```python
from build123d import *

# Parameters (mm, degrees)
PAD_DEPTH       = 12
POCKET_DEPTH    = 9
SKETCH002_R     = 2.1
POCKET001_DEPTH = 3
SKETCH003_R     = 1.6
POCKET002_DEPTH = 3.001
SKETCH004_R     = 3.2
POCKET003_DEPTH = 1


with BuildPart() as part:
    # Sketch → Pad (new body)
    with BuildSketch(Plane.XY):
        with BuildLine():
            ThreePointArc((10.4, 0), (0, 10.4), (-10.4, 0))
            Line((-10.4, 0), (-22.4, 0))
            Line((-22.4, 0), (-22.4, 3))
            Line((-22.4, 3), (-13.059862, 3))
            ThreePointArc((-4, 12.789058), (-9.834436, 9.10186), (-13.059862, 3))
            Line((-4, 12.789058), (-4, 22.789058))
            Line((-4, 22.789058), (4, 22.789058))
            Line((4, 22.789058), (4, 12.789058))
            ThreePointArc((13.059862, 3), (9.834436, 9.10186), (4, 12.789058))
            Line((22.4, 3), (13.059862, 3))
            Line((22.4, 0), (22.4, 3))
            Line((10.4, 0), (22.4, 0))
        make_face()
    extrude(amount=PAD_DEPTH)

    # Sketch001 (on Face14 of Pad) → Pocket (cut)
    with BuildSketch(Plane.XY.offset(12)):
        with BuildLine():
            Line((-4, 12.789058), (-4, 22.789058))
            Line((-4, 22.789058), (4, 22.789058))
            Line((4, 22.789058), (4, 12.789058))
            ThreePointArc((4, 12.789058), (0, 13.4), (-4, 12.789058))
        make_face()
    extrude(amount=-POCKET_DEPTH, mode=Mode.SUBTRACT)

    # Sketch002 (on Face16 of Pocket) → Pocket001 (cut)
    with BuildSketch(Plane.XY.offset(3)):
        with Locations((0, 18.094529)):
            Circle(SKETCH002_R)
    extrude(amount=-POCKET001_DEPTH, mode=Mode.SUBTRACT)

    # Sketch003 (on Face9 of Pocket001) → Pocket002 (cut, through all)
    with BuildSketch(Plane(origin=(0, 3, 0), x_dir=(-1, 0, 0), z_dir=(0, 1, 0))):
        with Locations((-17.729931, 6)):
            Circle(SKETCH003_R)
        with Locations((17.729931, 6)):
            Circle(SKETCH003_R)
    extrude(amount=-POCKET002_DEPTH, mode=Mode.SUBTRACT)

    # Sketch004 (on Face11 of Pocket002) → Pocket003 (cut)
    with BuildSketch(Plane(origin=(0, 3, 0), x_dir=(-1, 0, 0), z_dir=(0, 1, 0))):
        with Locations((-17.729931, 6)):
            Circle(SKETCH004_R)
        with Locations((17.729931, 6)):
            Circle(SKETCH004_R)
    extrude(amount=-POCKET003_DEPTH, mode=Mode.SUBTRACT)


solid = part.part
```
For this review, take the finished solid that the model builds, in its own axes (mm). A direction names the side the tool comes from. Give positions to 0.01 mm unless a question says otherwise; leave off trailing zeros. Order: outer loops, then holes, each group sorted by start corner. A loop starts at its lowest first (then second) coordinate and runs counter-clockwise, first axis right, second up.
1) Take a section at D-D (z = 10.25). Give the boundary of the cut face in (x, y), then the cut area to 3 significant figures.
2) Take a section at C-C (y = 17.25). Give the boundary of the cut face in (x, z).
3) Take a section at A-A (z = 6). Give the boundary of the cut face in (x, y), then the cut area to 3 significant figures.
4) The part is to be moulded in two halves that separate along Y. For faces 6 (the face through (22.4, 1, 6)), 7 (the face through (0.2, 10.4, 5.9)), 8 (the face through (0.97, 16.23, 1.52)), 9 (the face through (16, 2, 5)), say which applies: released by +Y, released by -Y, zero draft, split by the parting line, or undercut.
5) Take a section at B-B (x = 0). Give the boundary of the cut face in (y, z), then the cut area to 3 significant figures.
6) For faces 1 (the face through (4, 18, 1)), 2 (the face through (0, 11, 12)), 3 (the face through (-19.207, 2.507, 3.161)), 4 (the face through (-4, 18, 1)), 5 (the face through (-22.4, 1, 6)), list the 3-axis set-ups (+Z, -Z, +X, -X, +Y, -Y) from which the entire face can be reached by the end or side of a thin tool; tool diameter is ignored.
7) Wall thickness on line 1 (Y direction, x = 0, z = 1.15); line 2 (X direction, y = 6, z = 1); line 3 (Y direction, x = 0, z = 11.25): over which ranges is each line inside the solid? List them lowest first.
8) Insertion check: pin 1 (4.5 mm diameter, centred on x = 16.5, z = 8.5, fed in from +Y); pin 2 (1.5 mm diameter, centred on y = 19, z = 1.5, fed in from -X); pin 3 (2.5 mm diameter, centred on y = 20, z = 2, fed in from +X). Each pin has a flat end and moves straight along its axis. Give the tip position at first contact, or say it passes through.
Derived:
1. outline: (-22.4, 0) - (-10.4, 0) arc R10.4 cw to (10.4, 0) - (22.4, 0) - (22.4, 3) - (13.06, 3) arc R13.4 ccw to (4, 12.79) arc R13.4 ccw to (-4, 12.79) arc R13.4 ccw to (-13.06, 3) - (-22.4, 3) - close
1. area: 167 mm2
2. outline: (-4, 0) - (-1.92, 0) - (-1.92, 3) - (-4, 3) - close; (1.92, 0) - (4, 0) - (4, 3) - (1.92, 3) - close
3. outline: (-22.4, 0) - (-19.33, 0) - (-19.33, 2) - (-20.93, 2) - (-20.93, 3) - (-22.4, 3) - close; (-16.13, 0) - (-10.4, 0) arc R10.4 cw to (10.4, 0) - (16.13, 0) - (16.13, 2) - (14.53, 2) - (14.53, 3) - (13.06, 3) arc R13.4 ccw to (4, 12.79) arc R13.4 ccw to (-4, 12.79) arc R13.4 ccw to (-13.06, 3) - (-14.53, 3) - (-14.53, 2) - (-16.13, 2) - close; (19.33, 0) - (22.4, 0) - (22.4, 3) - (20.93, 3) - (20.93, 2) - (19.33, 2) - close
3. area: 141 mm2
4. face 6: zero draft
4. face 7: released by -Y
4. face 8: undercut
4. face 9: released by +Y
5. outline: (10.4, 0) - (15.99, 0) - (15.99, 3) - (13.4, 3) - (13.4, 12) - (10.4, 12) - close; (20.19, 0) - (22.79, 0) - (22.79, 3) - (20.19, 3) - close
5. area: 51.6 mm2
6. face 1: +Z, -Z, +X, +Y
6. face 2: +Z, +X, -X, +Y, -Y
6. face 3: +Y
6. face 4: +Z, -Z, -X, +Y
6. face 5: +Z, -Z, -X, +Y, -Y
7. line 1: y = 10.4 to 15.99, 20.19 to 22.79
7. line 2: x = -11.98 to -8.49, 8.49 to 11.98
7. line 3: y = 10.4 to 13.4
8. pin 1: stops at y = 3
8. pin 2: stops at x = -4
8. pin 3: stops at x = 4
